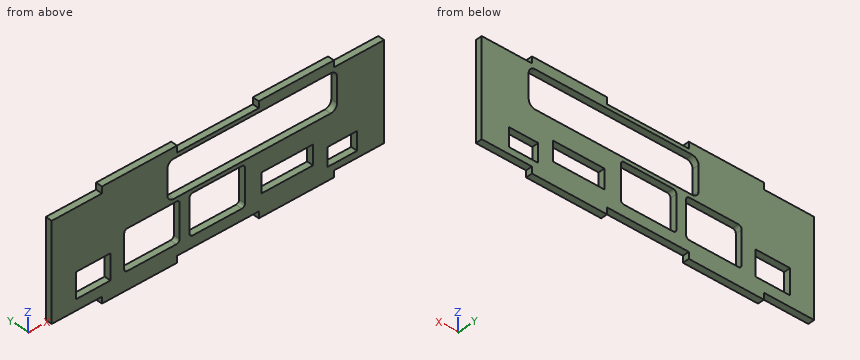
from build123d import *

# Parameters (mm, degrees)
SKETCH_1_W                     = 101.8
SKETCH_1_H                     = 29.5
EXTRUDE_1_DEPTH                = 2
SKETCH_2_W                     = 23
SKETCH_2_H                     = 2
EXTRUDE_2_DEPTH                = 2
SKETCH_3_W                     = 9
SKETCH_3_H                     = 5.7
CUT_EXTRUDE_1_DEPTH            = 3
SKETCH_4_W                     = 10.6
SKETCH_4_H                     = 7.8
CUT_EXTRUDE_2_DEPTH            = 3
SKETCH_6_W                     = 17
SKETCH_6_H                     = 12.2
CUT_EXTRUDE_4_DEPTH            = 3
FILLET_1_R                     = 1
PATTERN_LINEAR_1_COUNT         = 2
PATTERN_LINEAR_1_PITCH         = 20
FILLET_1_OF_PATTERN_LINEAR_1_R = 1
SKETCH_7_W                     = 15.8
SKETCH_7_H                     = 6
CUT_EXTRUDE_5_DEPTH            = 3
CUT_EXTRUDE_6_DEPTH            = 3


with BuildPart() as part:
    # 草图1 → 凸台-拉伸1 (new body)
    with BuildSketch(Plane(origin=(0, 0, 0), x_dir=(1, 0, 0), z_dir=(0, 1, 0))):
        Rectangle(SKETCH_1_W, SKETCH_1_H)
    extrude(amount=EXTRUDE_1_DEPTH)

    # 草图2 → 凸台-拉伸2 (add)
    with BuildSketch(Plane(origin=(0, 2, 0), x_dir=(1, 0, 0), z_dir=(0, 1, 0))):
        with Locations((-24, 15.75)):
            Rectangle(SKETCH_2_W, SKETCH_2_H)
        with Locations((24, 15.75)):
            Rectangle(SKETCH_2_W, SKETCH_2_H)
        with Locations((24, -15.75)):
            Rectangle(SKETCH_2_W, SKETCH_2_H)
        with Locations((-24, -15.75)):
            Rectangle(SKETCH_2_W, SKETCH_2_H)
    extrude(amount=-EXTRUDE_2_DEPTH)

    # 草图3 → 切除-拉伸1 (cut, through all)
    with BuildSketch(Plane(origin=(0, 2, 0), x_dir=(1, 0, 0), z_dir=(0, 1, 0))):
        with Locations((38.1, 9.9)):
            Rectangle(SKETCH_3_W, SKETCH_3_H)
    extrude(amount=-CUT_EXTRUDE_1_DEPTH, mode=Mode.SUBTRACT)

    # 草图4 → 切除-拉伸2 (cut, through all)
    with BuildSketch(Plane(origin=(0, 2, 0), x_dir=(1, 0, 0), z_dir=(0, 1, 0))):
        with Locations((-38.2, 7.55)):
            Rectangle(SKETCH_4_W, SKETCH_4_H)
    extrude(amount=-CUT_EXTRUDE_2_DEPTH, mode=Mode.SUBTRACT)

    # 草图6 → 切除-拉伸4 (cut, through all)
    with BuildSketch(Plane(origin=(0, 2, 0), x_dir=(1, 0, 0), z_dir=(0, 1, 0))):
        with Locations((-20.2, 5.25)):
            Rectangle(SKETCH_6_W, SKETCH_6_H)
    cut_extrude_4 = extrude(amount=-CUT_EXTRUDE_4_DEPTH, mode=Mode.SUBTRACT)

    # 圆角1
    fillet_1_edges = [part.edges().sort_by_distance(p)[0] for p in [
        (-28.7, 1, 0.85),
        (-28.7, 1, -11.35),
        (-11.7, 1, -11.35),
        (-11.7, 1, 0.85),
    ]]
    fillet(fillet_1_edges, radius=FILLET_1_R)

    # 阵列(线性)1: 切除-拉伸4 ×2
    with Locations(*[(i * PATTERN_LINEAR_1_PITCH, 0, 0) for i in range(1, PATTERN_LINEAR_1_COUNT)]):
        add(cut_extrude_4, mode=Mode.SUBTRACT)

    # 圆角1 of 阵列(线性)1
    fillet_1_of_pattern_linear_1_edges = [part.edges().sort_by_distance(p)[0] for p in [
        (-8.7, 1, 0.85),
        (-8.7, 1, -11.35),
        (8.3, 1, -11.35),
        (8.3, 1, 0.85),
    ]]
    fillet(fillet_1_of_pattern_linear_1_edges, radius=FILLET_1_OF_PATTERN_LINEAR_1_R)

    # 草图7 → 切除-拉伸5 (cut, through all)
    with BuildSketch(Plane(origin=(0, 2, 0), x_dir=(1, 0, 0), z_dir=(0, 1, 0))):
        with Locations((21.2, 7.05)):
            Rectangle(SKETCH_7_W, SKETCH_7_H)
    extrude(amount=-CUT_EXTRUDE_5_DEPTH, mode=Mode.SUBTRACT)

    # 草图8 → 切除-拉伸6 (cut, through all)
    with BuildSketch(Plane(origin=(0, 2, 0), x_dir=(1, 0, 0), z_dir=(0, 1, 0))):
        with BuildLine():
            Line((-13.5, -2.05), (34.5, -2.05))
            ThreePointArc((34.5, -2.05), (35.914213562, -2.635786438), (36.5, -4.05))
            Line((36.5, -4.05), (36.5, -11.55))
            ThreePointArc((36.5, -11.55), (35.914213562, -12.964213562), (34.5, -13.55))
            Line((34.5, -13.55), (-13.5, -13.55))
            ThreePointArc((-13.5, -13.55), (-14.914213562, -12.964213562), (-15.5, -11.55))
            Line((-15.5, -11.55), (-15.5, -4.05))
            ThreePointArc((-15.5, -4.05), (-14.914213562, -2.635786438), (-13.5, -2.05))
        make_face()
    extrude(amount=-CUT_EXTRUDE_6_DEPTH, mode=Mode.SUBTRACT)


solid = part.part
Input: part model. Units: mm. Frame: model coordinates. Give positions to 0.01 mm unless a question says otherwise; leave off trailing zeros. Write each loop counter-clockwise with the first axis right and the second up, starting at its lowest first coordinate (ties: lowest second). Pieces come first, ordered by that corner, then holes. Notation, with made-up numbers: M -18,-37 L 6,-37 A21 ccw 6,-9 Z; hole C -34,66 d1. An arc over 180 degrees is marked long. Use one line per item in the form item = value.
1. Cut plane C-C on x = -34. Return loops of the section in (y, z).
Outcome:
outline = M 0,-16.75 L 2,-16.75 L 2,-11.45 L 0,-11.45 Z; M 0,-3.65 L 2,-3.65 L 2,16.75 L 0,16.75 Z
2. Cut plane B-B on z = -5. Return loops of the section in (x, y), and give its area (3 significant figures).
Outcome:
outline = M -50.9,0 L -43.5,0 L -43.5,2 L -50.9,2 Z; M -32.9,0 L -28.7,0 L -28.7,2 L -32.9,2 Z; M -11.7,0 L -8.7,0 L -8.7,2 L -11.7,2 Z; M 8.3,0 L 13.3,0 L 13.3,2 L 8.3,2 Z; M 29.1,0 L 50.9,0 L 50.9,2 L 29.1,2 Z
area = 82.8 mm²
3. Cut plane A-A on x = 16. Return loops of the section in (y, z).
Outcome:
outline = M 0,-16.75 L 2,-16.75 L 2,-10.05 L 0,-10.05 Z; M 0,-4.05 L 2,-4.05 L 2,2.05 L 0,2.05 Z; M 0,13.55 L 2,13.55 L 2,16.75 L 0,16.75 Z
4. Cut plane D-D on y = 1.65. State how many separate pieces and enclosed holes the cut face has, and give its area (3 significant figures).
Outcome:
separate_pieces = 1
enclosed_holes = 6
area = 1,950 mm²
5. First-contact query: P1, Ø0.6, axis at x = -36.5, y = 1, coming from the -Z side. Flat tip, straight axial feed; report the tip coordinate or a pass-through.
Outcome:
P1 = -14.75
6. Ray query, L1, parallel to Z at x = 1.5, y = 1.95; L2, parallel to X at y = 1.3, z = -9; L3, parallel to X at y = 1.3, z = -4.5. Return the intervals inside material, ascending.
Outcome:
L1 = -14.75 to -11.35, 0.85 to 2.05, 13.55 to 14.75
L2 = -50.9 to -43.5, -32.9 to -28.7, -11.7 to -8.7, 8.3 to 13.3, 29.1 to 33.6, 42.6 to 50.9
L3 = -50.9 to -43.5, -32.9 to -28.7, -11.7 to -8.7, 8.3 to 13.3, 29.1 to 50.9
